Geometry: see drawing. Coordinates: mm, zero at the bounding-box minimum. A direction names the side the tool comes from. Give positions to 0.01 mm unless a question says otherwise; leave off trailing zeros. Loops run counter-clockwise (first coordinate to the right, second up) from the corner with the lowest first, then second, coordinate; pieces in that order, holes last. Notation, with made-up numbers: M 45.5,54 L 53.5,54 A20 ccw 53.5,93 Z; hole C 77.5,44 d7. An arc over 180 degrees is marked long. Answer in a Markdown table with one row per item.
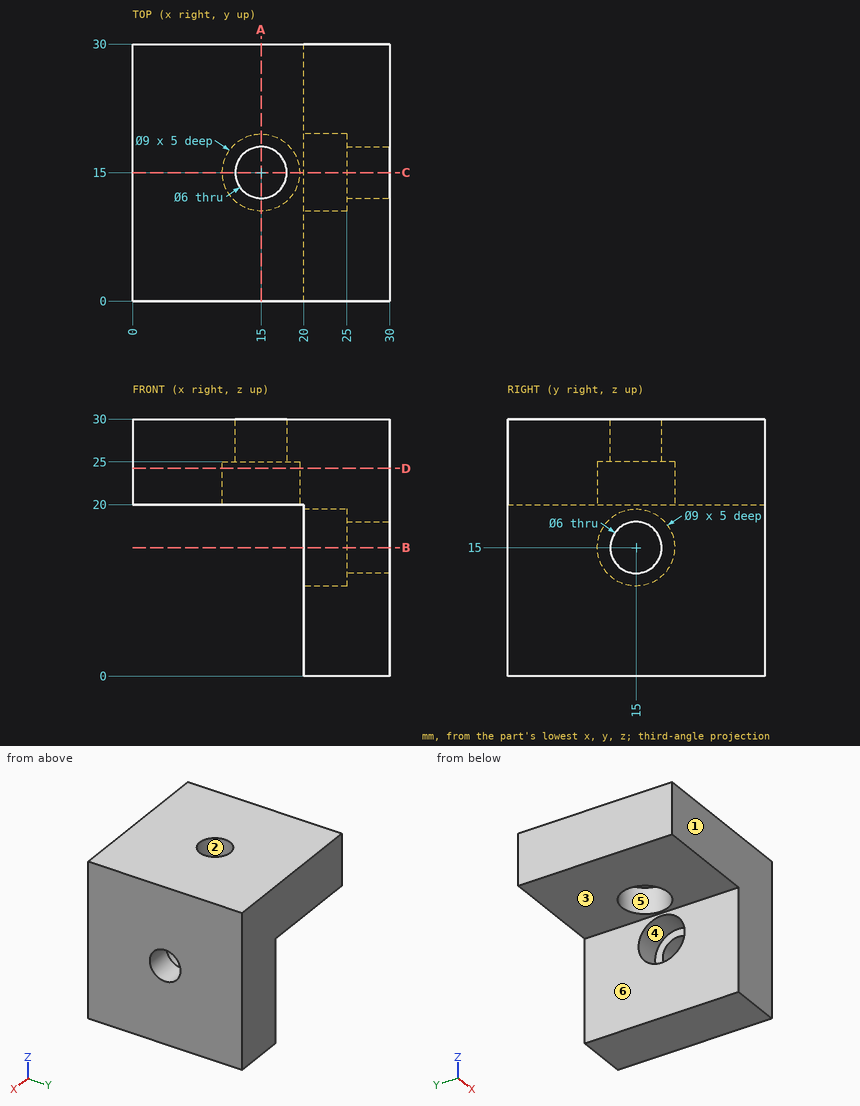
1) Section D-D, the plane z = 24.25. Return loops of the section in (x, y), then the cut area to 3 significant figures.
Reply:
| item | result |
|---|---|
| outline | M 0,0 L 30,0 L 30,30 L 0,30 Z; hole C 15,15 d9 |
| area | 836 mm² |
2) Section A-A, the plane x = 15. Return loops of the section in (y, z), then the cut area to 3 significant figures.
Reply:
| item | result |
|---|---|
| outline | M 0,20 L 10.5,20 L 10.5,25 L 12,25 L 12,30 L 0,30 Z; M 18,25 L 19.5,25 L 19.5,20 L 30,20 L 30,30 L 18,30 Z |
| area | 225 mm² |
3) Section C-C, the plane y = 15. Return loops of the section in (x, z).
Reply:
| item | result |
|---|---|
| outline | M 0,20 L 10.5,20 L 10.5,25 L 12,25 L 12,30 L 0,30 Z; M 18,25 L 19.5,25 L 19.5,20 L 20,20 L 20,19.5 L 25,19.5 L 25,18 L 30,18 L 30,30 L 18,30 Z; M 20,0 L 30,0 L 30,12 L 25,12 L 25,10.5 L 20,10.5 Z |
4) Pull-direction query (Y, two-part tool) for the marked faces 1, 2 and 3; classes: released by +Y, released by -Y, zero draft, split by the parting line, or undercut.
Reply:
| item | result |
|---|---|
| face 1 | released by -Y |
| face 2 | undercut |
| face 3 | zero draft |
5) Material intervals for L1, parallel to Y at x = 27.5, z = 15; L2, parallel to Z at x = 4, y = 27.25, sorted ascending.
Reply:
| item | result |
|---|---|
| L1 | y = 0 to 12, 18 to 30 |
| L2 | z = 20 to 30 |
6) Pin query (flat end, axial travel): pin 1 Ø3 at (y, z) = (15.5, 4) entering from -X; pin 2 Ø4.5 at (y, z) = (16, 15.5) entering from -X; pin 3 Ø5 at (x, y) = (11, 9) entering from -Z. Return the tip coordinate at first contact, or that it passes through.
Reply:
| item | result |
|---|---|
| pin 1 | stops at x = 20 |
| pin 2 | stops at x = 25 |
| pin 3 | stops at z = 20 |
7) Section B-B, the plane z = 15. Return loops of the section in (x, y), then the cut area to 3 significant figures.
Reply:
| item | result |
|---|---|
| outline | M 20,0 L 30,0 L 30,12 L 25,12 L 25,10.5 L 20,10.5 Z; M 20,19.5 L 25,19.5 L 25,18 L 30,18 L 30,30 L 20,30 Z |
| area | 225 mm² |
8) Set-up query: the marked faces 4, 5 and 6. Return all of +Z, -Z, +X, -X, +Y, -Y with unobstructed straight access to the full face (end or side cutting, diameter ignored); none if empty.
Reply:
| item | result |
|---|---|
| face 4 | -X |
| face 5 | -Z |
| face 6 | -Z, -X, +Y, -Y |
